```python
from build123d import *

# Parameters (mm, degrees)
SKETCH_W        = 170
SKETCH_H        = 15
PAD_DEPTH       = 10
SKETCH001_W     = 35
SKETCH001_H     = 25
POCKET_DEPTH    = 5
SKETCH002_R     = 5
PAD001_DEPTH    = 5
PAD002_DEPTH    = 10
POCKET001_DEPTH = 10
SKETCH005_W     = 15.25
SKETCH005_H     = 10
PAD003_DEPTH    = 2.5


with BuildPart() as part:
    # Sketch → Pad (new body)
    with BuildSketch(Plane.XY):
        with Locations((-20.728933, -1.58076)):
            Rectangle(SKETCH_W, SKETCH_H)
    extrude(amount=PAD_DEPTH)

    # Sketch001 (on Face6 of Pad) → Pocket (cut)
    with BuildSketch(Plane.XY.offset(10)):
        with Locations((51.771067, -1.58076)):
            Rectangle(SKETCH001_W, SKETCH001_H)
    extrude(amount=-POCKET_DEPTH, mode=Mode.SUBTRACT)

    # Sketch002 (on Face7 of Pocket) → Pad001 (join)
    with BuildSketch(Plane.XY.offset(5)):
        with Locations((56.771067, -1.58076)):
            Circle(SKETCH002_R)
        with Locations((41.771067, -1.58076)):
            Circle(SKETCH002_R)
    extrude(amount=PAD001_DEPTH)

    # Sketch003 (on Face1 of Pad001) → Pad002 (join)
    with BuildSketch(Plane(origin=(-105.728933, 0, 0), x_dir=(0, -1, 0), z_dir=(-1, 0, 0))):
        Polygon((-5.91924, 0), (-0.145737, 10), (3.307257, 10), (9.08076, 0), align=None)
    extrude(amount=PAD002_DEPTH)

    # Sketch004 (on Face3 of Pad002) → Pocket001 (cut)
    with BuildSketch(Plane.XY.offset(10)):
        Polygon((-93.103933, -14.787648), (-100.728933, -1.58076), (-85.478933, -1.58076), align=None)
    extrude(amount=-POCKET001_DEPTH, mode=Mode.SUBTRACT)

    # Sketch005 (on Face9 of Pocket001) → Pad003 (join)
    with BuildSketch(Plane(origin=(0, 5.91924, 0), x_dir=(-1, 0, 0), z_dir=(0, 1, 0))):
        with Locations((93.103933, 5)):
            Rectangle(SKETCH005_W, SKETCH005_H)
    extrude(amount=PAD003_DEPTH)


solid = part.part
```
Can you work these out from the model? Positions are in its coordinate system, mm. A direction names the side the tool comes from. Coordinates: 2 decimals unless noted, no trailing zeros. Loops run counter-clockwise (first coordinate to the right, second up) from the corner with the lowest first, then second, coordinate; pieces in that order, holes last. Notation, with made-up numbers: (76.25, 60.25) - (116.25, 60.25) arc R13 ccw to (116.25, 81.25) - close; hole circle Ø8 at (45, 2.25). An arc over 180 degrees is marked (long way). Use a Markdown table: item, result.
Item 1: If I drill on probe 1 along X at (y, z) = (-3, 7.5); probe 2 along X at (y, z) = (0.5, 8.25); probe 3 along X at (y, z) = (5.5, 1), over which ranges is the centre line in solid material (lowest first)? Write a range as from..to.
Numbers:
| item | result |
|---|---|
| probe 1 | x = -115.73..-99.91, -86.3..34.27, 36.98..46.57, 51.98..61.57 |
| probe 2 | x = -115.73..34.27, 37.22..46.32, 52.22..61.32 |
| probe 3 | x = -105.73..64.27 |
Item 2: We'd pull the mould along X, two halves only. Please class faces 4 (the face through (-87.614, -5.278, 5.07)), 5 (the face through (42, -2, 10)), 6 (the face through (-105.729, 4, 7)), 7 (the face through (-93, -1.581, 5)): released by +X, released by -X, zero draft, split by the parting line, or undercut.
Numbers:
| item | result |
|---|---|
| face 4 | undercut |
| face 5 | zero draft |
| face 6 | released by -X |
| face 7 | undercut |
Item 3: I want a section at C-C on x = 44. Please give me the cut outline in (y, z).
Numbers:
| item | result |
|---|---|
| outline | (-9.08, 0) - (5.92, 0) - (5.92, 5) - (2.89, 5) - (2.89, 10) - (-6.06, 10) - (-6.06, 5) - (-9.08, 5) - close |
Item 4: For faces 1 (the face through (-110.659, -6.154, 5.07)), 2 (the face through (-98.534, -5.383, 5.07)), 3 (the face through (46.39, -3.5, 7.46)), which set-ups out of +Z, -Z, +X, -X, +Y, -Y let a thin tool reach every point of the face, with its end or its side?
Numbers:
| item | result |
|---|---|
| face 1 | +Z, -X, -Y |
| face 2 | +Z, -Z |
| face 3 | +Z |
Item 5: Will these pins go through, and if not, where does the flat tip stop? pin 1 (6 mm diameter, centred on x = -17, z = 8.5, fed in from +Y); pin 2 (1.2 mm diameter, centred on y = 7.5, z = 4.5, fed in from +X); pin 3 (1.2 mm diameter, centred on y = 7.5, z = 5, fed in from -X).
Numbers:
| item | result |
|---|---|
| pin 1 | stops at y = 5.92 |
| pin 2 | stops at x = -85.48 |
| pin 3 | stops at x = -100.73 |
Item 6: I want a section at B-B on x = 24. Please give me the cut outline in (y, z).
Numbers:
| item | result |
|---|---|
| outline | (-9.08, 0) - (5.92, 0) - (5.92, 10) - (-9.08, 10) - close |
Item 7: I want a section at A-A on z = 8. Please give me the cut outline in (x, y).
Numbers:
| item | result |
|---|---|
| outline | (-115.73, -4.46) - (-105.73, -4.46) - (-105.73, -9.08) - (-96.4, -9.08) - (-100.73, -1.58) - (-85.48, -1.58) - (-89.81, -9.08) - (34.27, -9.08) - (34.27, 5.92) - (-85.48, 5.92) - (-85.48, 8.42) - (-100.73, 8.42) - (-100.73, 5.92) - (-105.73, 5.92) - (-105.73, 1.3) - (-115.73, 1.3) - close; circle Ø10 at (41.77, -1.58); circle Ø10 at (56.77, -1.58) |
